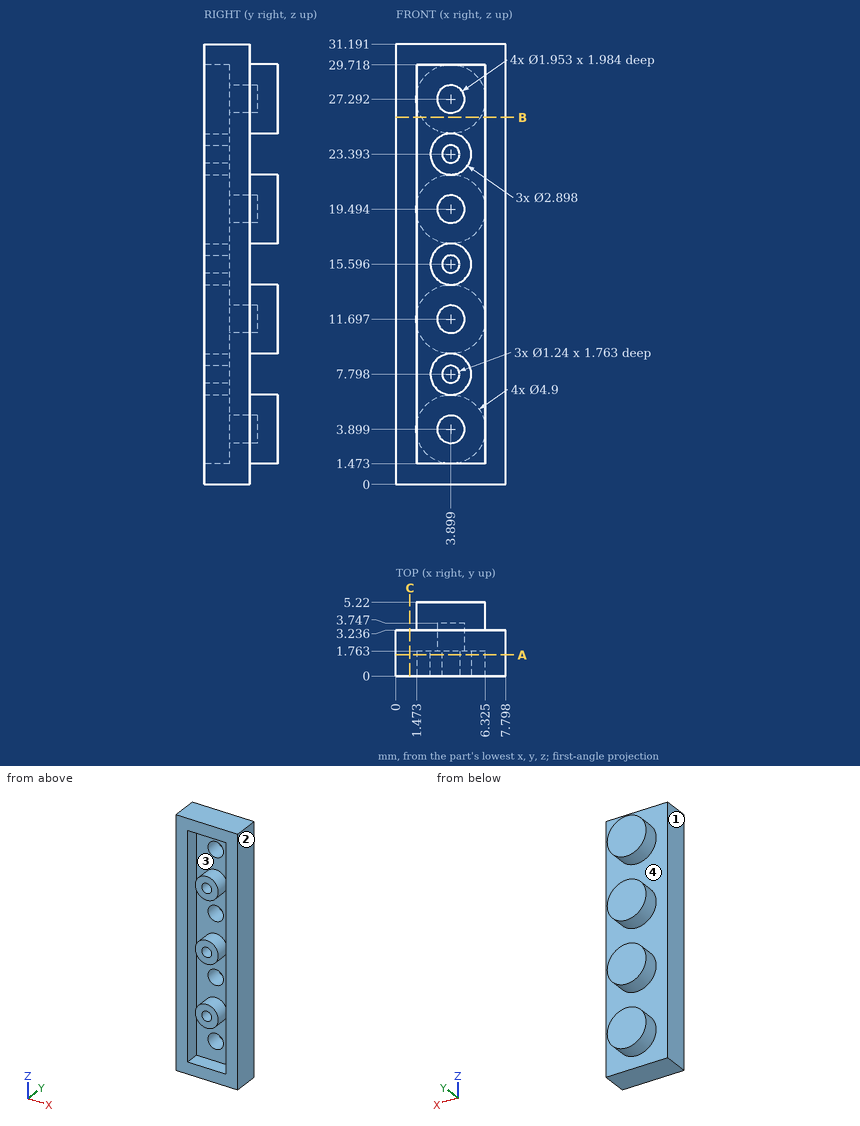
The figure shows three views and two pictorial views of one solid part (mm, origin at its lowest corner). Answer the questions. Coordinates: 2 decimals unless noted, no trailing zeros. Write each loop counter-clockwise with the first axis right and the second up, starting at its lowest first coordinate (ties: lowest second). Pieces come first, ordered by that corner, then holes. Notation, with made-up numbers: (79.25, 48) -> (98.25, 48) arc R28 cw to (98.25, 83) -> close; hole circle Ø7 at (71.25, 84.25). An arc over 180 degrees is marked (long way). Return JSON: item names as keys, results as strings.
(1) Each of these flat-tipped pins is pushed along its axis until it touches: P1, Ø3, axis at y = 1, z = 26.5, coming from the -X side; P2, Ø1.1, axis at x = 3.9, z = 23.39, coming from the -Y side; P3, Ø0.6, axis at x = 4, z = 12, coming from the -Y side; P4, Ø1.5, axis at x = 1.5, z = 23, coming from the +Y side. Where does it stop, or does it pass through?
Answers below:
{"P1": "x = 0", "P2": "y = 1.76", "P3": "y = 3.75", "P4": "y = 3.24"}
(2) For a pull along X with two mould halves and no side action, classify the marked faces 1, 2, 3 and 4 as pulls with the +X half, pulls with the -X half, needs draft (parallel to the pull), parting line crosses it, or undercut.
Answers below:
{"face 1": "pulls with the -X half", "face 2": "pulls with the +X half", "face 3": "undercut", "face 4": "needs draft"}
(3) Consider line 1 along X through (y, z) = (0.45, 6) (1 decimal); line 2 along X through (y, z) = (0.9, 15.5) (1 decimal); line 3 along Z through (x, y) = (3.25, 4) (1 decimal). Determine where each line is inside the solid, lowest interval first. Write a range as from..to.
Answers below:
{"line 1": "0..1.5, 6.3..7.8", "line 2": "0..1.5, 2.5..3.3, 4.5..5.3, 6.3..7.8", "line 3": "1.5..6.3, 9.3..14.1, 17.1..21.9, 24.9..29.7"}
(4) The part is cut by section C-C on x = 1. Give the vertices of the cut face in (y, z) (1 decimal), then the cut area to 3 significant figures.
Answers below:
{"outline": "(0, 0) -> (3.2, 0) -> (3.2, 31.2) -> (0, 31.2) -> close", "area": "101 mm^2"}
(5) The part is cut by section A-A on y = 1.5. State how many separate pieces and enclosed holes the cut face has.
Answers below:
{"separate pieces": "4", "enclosed holes": "4"}
(6) The part is cut by section B-B on z = 26. Give the vertices of the cut face in (x, y) (1 decimal).
Answers below:
{"outline": "(0, 0) -> (1.5, 0) -> (1.5, 1.8) -> (6.3, 1.8) -> (6.3, 0) -> (7.8, 0) -> (7.8, 3.2) -> (6, 3.2) -> (6, 5.2) -> (1.8, 5.2) -> (1.8, 3.2) -> (0, 3.2) -> close"}
